Could you check a few things on this drawing? It's one solid part, dimensions in mm from its lowest x, y, z. A direction names the side the tool comes from. Give positions to 0.01 mm unless a question says otherwise; leave off trailing zeros. Order: outer loops, then holes, each group sorted by start corner. A loop starts at its lowest first (then second) coordinate and runs counter-clockwise, first axis right, second up.
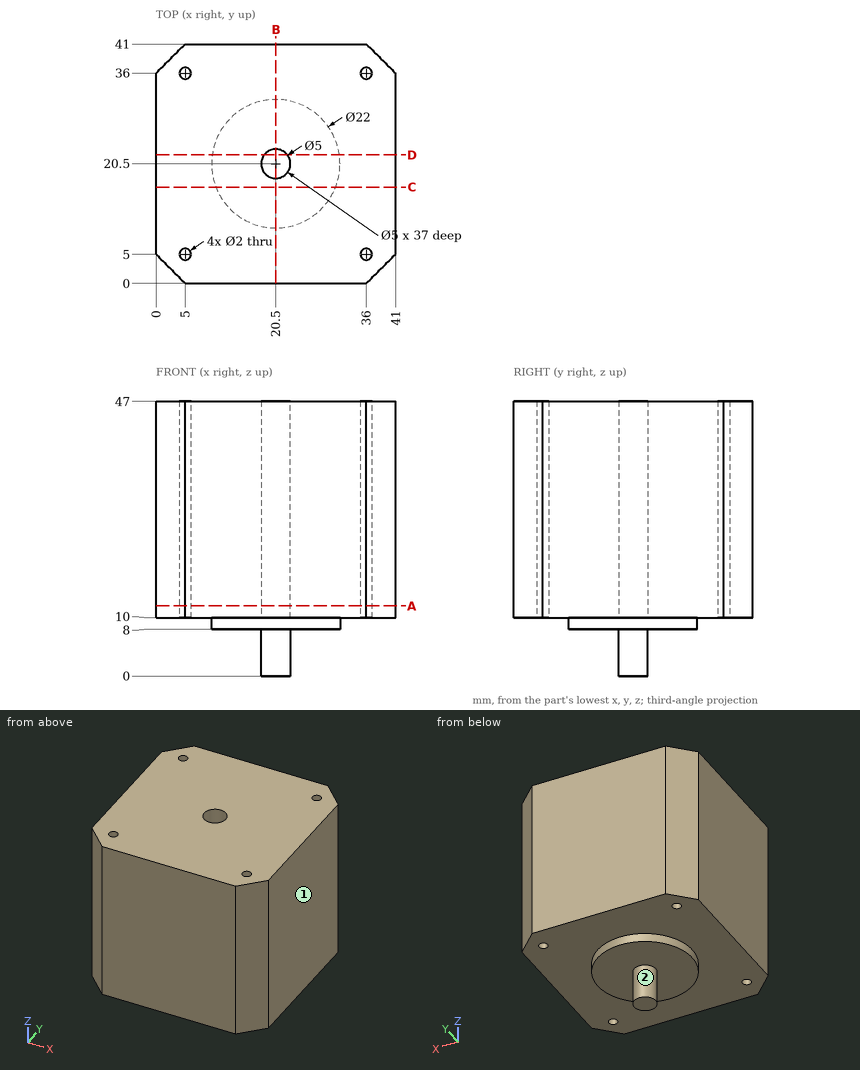
Item 1: For pin 1 (4 mm diameter, centred on y = 27, z = 6.5, fed in from +X); pin 2 (2.5 mm diameter, centred on x = 21.5, y = 21, fed in from +Z); pin 3 (1.2 mm diameter, centred on x = 5, y = 36, fed in from +Z), each with a flat end and sliding along its axis, tell me the tip position at first contact or that it passes through.
Findings:
pin 1: stops at x = 30.21
pin 2: stops at z = 10
pin 3: passes through
Item 2: Imagine slicing it at D-D on y = 22. List the corners of the cut face in (x, z) for me, then the cut area to 3 significant figures.
Findings:
outline: (0, 10) - (9.6, 10) - (9.6, 8) - (18.5, 8) - (18.5, 0) - (22.5, 0) - (22.5, 8) - (31.4, 8) - (31.4, 10) - (41, 10) - (41, 47) - (22.5, 47) - (22.5, 10) - (18.5, 10) - (18.5, 47) - (0, 47) - close
area: 1,440 mm2
Item 3: Imagine slicing it at A-A on z = 12. List the corners of the cut face in (x, y) for me.
Findings:
outline: (0, 5) - (5, 0) - (36, 0) - (41, 5) - (41, 36) - (36, 41) - (5, 41) - (0, 36) - close; hole circle Ø2 at (5, 5); hole circle Ø2 at (5, 36); hole circle Ø5 at (20.5, 20.5); hole circle Ø2 at (36, 5); hole circle Ø2 at (36, 36)
Item 4: For the marked faces 1 and 2, which set-ups out of +Z, -Z, +X, -X, +Y, -Y let a thin tool reach every point of the face, with its end or its side?
Findings:
face 1: +Z, -Z, +X, +Y, -Y
face 2: -Z
Item 5: Please list where these lines run through material, in increasing order: line 1 along Y through (x, z) = (36, 24); line 2 along Z through (x, y) = (19.5, 17); line 3 along Z through (x, y) = (38, 24).
Findings:
line 1: y = 0 to 4, 6 to 35, 37 to 41
line 2: z = 8 to 47
line 3: z = 10 to 47
Item 6: Imagine slicing it at C-C on y = 16.5. List the corners of the cut face in (x, z) for me, then the cut area to 3 significant figures.
Findings:
outline: (0, 10) - (10.25, 10) - (10.25, 8) - (30.75, 8) - (30.75, 10) - (41, 10) - (41, 47) - (0, 47) - close
area: 1,560 mm2
Item 7: Imagine slicing it at B-B on x = 20.5. List the corners of the cut face in (y, z) for me.
Findings:
outline: (0, 10) - (9.5, 10) - (9.5, 8) - (18, 8) - (18, 0) - (23, 0) - (23, 8) - (31.5, 8) - (31.5, 10) - (41, 10) - (41, 47) - (23, 47) - (23, 10) - (18, 10) - (18, 47) - (0, 47) - close
